Source: CAD feature listing. Evaluate the final solid. Frame: model axes, mm. A direction names the side the tool comes from. Give positions to 0.01 mm unless a question says otherwise; leave off trailing zeros. Loops run counter-clockwise (first coordinate to the right, second up) from the corner with the lowest first, then second, coordinate; pieces in that order, holes last. Notation, with made-up numbers: M 81,19 L 133,19 A23 ccw 133,38 Z; hole C 79.25,-23 d8. An arc over 180 degrees is marked long. Answer in a Markdown table with one row per item.
```python
from build123d import *

# Parameters (mm, degrees)
SKETCH2_R           = 7.5
BOSS_EXTRUDE1_DEPTH = 10
SKETCH3_R           = 15
SKETCH3_R_2         = 7.5
BOSS_EXTRUDE2_DEPTH = 20


with BuildPart() as part:
    # Sketch2 → Boss-Extrude1 (new body)
    with BuildSketch(Plane(origin=(0, 0, 0), x_dir=(1, 0, 0), z_dir=(0, 1, 0))):
        with BuildLine():
            Line((-230, 25), (0, 25))
            ThreePointArc((0, 25), (25, 0), (0, -25))
            Line((0, -25), (-230, -25))
            ThreePointArc((-230, -25), (-255, 0), (-230, 25))
        make_face()
        with Locations(Location((-230, 0, 0), (0, 0, 270))):
            Circle(SKETCH2_R, mode=Mode.SUBTRACT)
        with BuildLine():
            Line((-190, 10), (0, 10))
            ThreePointArc((0, 10), (10, 0), (0, -10))
            Line((0, -10), (-190, -10))
            Line((-190, -10), (-200, -10))
            ThreePointArc((-200, -10), (-210, 0), (-200, 10))
            Line((-200, 10), (-190, 10))
        make_face(mode=Mode.SUBTRACT)
    extrude(amount=BOSS_EXTRUDE1_DEPTH)

    # Sketch3 → Boss-Extrude2 (add)
    with BuildSketch(Plane.XZ):
        with Locations(Location((-230, 0, 0), (0, 0, 270))):
            Circle(SKETCH3_R)
        with Locations(Location((-230, 0, 0), (0, 0, 270))):
            Circle(SKETCH3_R_2, mode=Mode.SUBTRACT)
    extrude(amount=-BOSS_EXTRUDE2_DEPTH)


solid = part.part
```
Q1. Section query A-A (x = -72). Output: boundary loops of the cut face in (y, z).
Values follow:
| item | result |
|---|---|
| outline | M 0,-25 L 10,-25 L 10,-10 L 0,-10 Z; M 0,10 L 10,10 L 10,25 L 0,25 Z |
Q2. Contact query for flat-ended pins moving along their axis: pin 1 Ø2 at (y, z) = (18, -10.5) entering from -X; pin 2 Ø8 at (y, z) = (15, 12) entering from +X; pin 3 Ø5 at (x, y) = (-63, 12) entering from -Z; pin 4 Ø12 at (y, z) = (17, 0.5) entering from +X. Output: stop coordinate, or through.
Values follow:
| item | result |
|---|---|
| pin 1 | x = -241.61 |
| pin 2 | x = -217.31 |
| pin 3 | z = -25 |
| pin 4 | x = -215 |
Q3. Section query B-B (z = 0). Output: boundary loops of the cut face in (x, y), plus the area to 3 significant figures.
Values follow:
| item | result |
|---|---|
| outline | M -255,0 L -237.5,0 L -237.5,20 L -245,20 L -245,10 L -255,10 Z; M -222.5,0 L -210,0 L -210,10 L -215,10 L -215,20 L -222.5,20 Z; M 10,0 L 25,0 L 25,10 L 10,10 Z |
| area | 600 mm^2 |
Q4. Section query D-D (x = -234). Output: boundary loops of the cut face in (y, z).
Values follow:
| item | result |
|---|---|
| outline | M 0,-24.68 L 10,-24.68 L 10,-14.46 L 20,-14.46 L 20,-6.34 L 0,-6.34 Z; M 0,6.34 L 20,6.34 L 20,14.46 L 10,14.46 L 10,24.68 L 0,24.68 Z |
Q5. Section query C-C (y = 6.75). Output: boundary loops of the cut face in (x, z), plus the area to 3 significant figures.
Values follow:
| item | result |
|---|---|
| outline | M -230,-25 L 0,-25 A25 ccw 0,25 L -230,25 A25 ccw Z; hole C -230,0 d15; hole M -200,-10 L 0,-10 A10 ccw 0,10 L -200,10 A10 ccw Z |
| area | 8,970 mm^2 |
Q6. Reachability of faces 5 (the cylindrical face through (-244.643, 14.93, 3.252)), 6 (the flat face through (-99, 5, 10)), 7 (the flat face through (-113, 5, 25)) from +Z, -Z, +X, -X, +Y, -Y: full face, straight path, thin tool, end or side. Return the list, or none.
Values follow:
| item | result |
|---|---|
| face 5 | +Y |
| face 6 | +Y, -Y |
| face 7 | +Z, +X, -X, +Y, -Y |
Q7. Ray query, probe 1 along Z at (x, y) = (-131, 6.75); probe 2 along X at (y, z) = (12.75, 0); probe 3 along Y at (x, z) = (8.5, 22). Return the intervals inside material, ascending. Write a range as from..to.
Values follow:
| item | result |
|---|---|
| probe 1 | -25..-10, 10..25 |
| probe 2 | -245..-237.5, -222.5..-215 |
| probe 3 | 0..10 |
Q8. Mould query, pull axis X, two halves, no side actions, for faces 1 (the cylindrical face through (24.994, 4.93, -0.55)), 2 (the cylindrical face through (-210, 5, 0)), 3 (the flat face through (-101, 5, -10)), 4 (the flat face through (-117, 5, -25)). Classes: +X half, -X half, draft (parallel to the pull), parting line (faces both ways), or undercut.
Values follow:
| item | result |
|---|---|
| face 1 | +X half |
| face 2 | undercut |
| face 3 | undercut |
| face 4 | draft |
